from build123d import *

# Parameters (mm, degrees)
F1_DEPTH = 76.2
F2_T     = -2.54


with BuildPart() as f1:
    # F0 (on Top) → F1 (new body)
    with BuildSketch(Plane.XY):
        Polygon((43.9940905122, 25.4), (21.9970452561, 12.7), (21.9970452561, -12.7), (43.9940905122, -25.4), (65.9911357684, -12.7), (65.9911357684, 12.7), align=None)
        Polygon((0, 25.4), (21.9970452561, 12.7), (43.9940905122, 25.4), (43.994090537, 50.8000000143), (21.9970452561, 63.5000000285), (-2.47e-08, 50.8000000143), align=None)
        Polygon((43.9940905122, -25.4), (21.9970452561, -12.7), (0, -25.4), (0, -50.8), (21.9970452561, -63.5), (43.9940905122, -50.8), align=None)
        Polygon((-21.9970452561, 12.7), (0, 25.4), (0, 50.8), (-21.9970452561, 63.5), (-43.9940905122, 50.8), (-43.9940905122, 25.4), align=None)
        Polygon((0, -50.8), (0, -25.4), (-21.9970452561, -12.7), (-43.9940905122, -25.4), (-43.9940905122, -50.8), (-21.9970452561, -63.5), align=None)
        Polygon((-21.9970452561, -12.7), (-21.9970452561, 12.7), (-43.9940905122, 25.4), (-65.9911357684, 12.7), (-65.9911357684, -12.7), (-43.9940905122, -25.4), align=None)
        Polygon((21.9970452561, -12.7), (21.9970452561, 12.7), (0, 25.4), (-21.9970452561, 12.7), (-21.9970452561, -12.7), (0, -25.4), align=None)
    extrude(amount=F1_DEPTH)

    # F2
    f2_openings = [f1.faces().sort_by_distance(p)[0] for p in [
        (0, 0, 76.2),
    ]]
    offset(amount=F2_T, openings=f2_openings, kind=Kind.INTERSECTION)


solid = f1.part
Geometry check sheet. Reference: the model listing, model coordinates, mm. A direction names the side the tool comes from. Round coordinates to 2 decimals unless told otherwise and drop trailing zeros. Loops run counter-clockwise (first coordinate to the right, second up) from the corner with the lowest first, then second, coordinate; pieces in that order, holes last. Notation, with made-up numbers: (20.5, -29.5) - (31.5, -29.5) arc R23 cw to (31.5, -5.5) - close; hole circle Ø2 at (7.5, 33). An arc over 180 degrees is marked (long way). One line per question, with ' | ' between items. Start each with the question number.
1. Scan lines: line 1 (X direction, y = 8, z = 13); line 2 (X direction, y = -46, z = 64); line 3 (Z direction, x = -11.5, y = -26.5). Record each from-to range of solid material in increasing order. Write a range as [from, to].
2. Draft check along Y on faces 1 (the face through (-33.15, -57.06, 37.57)), 2 (the face through (-52.3, 17.67, 38.85)), 3 (the face through (-43.994, -38, 38)). Enter one of: released by +Y, released by -Y, zero draft, split by the parting line, or undercut.
3. Depth check by flat-ended pin: pin 1 (12.5 mm diameter, centred on y = -33, z = 38.5, fed in from +X); pin 2 (4 mm diameter, centred on x = 30, y = 50, fed in from +Z); pin 3 (5 mm diameter, centred on x = 36.5, z = 64.5, fed in from +Y). Enter the tip coordinate at first touch or a pass-through.
4. Tool access check on faces 4 (the face through (-43.994, 38, 38)), 5 (the face through (-11.153, -57.239, 37.567)), 6 (the face through (-10.84, 57.06, 37.57)), 7 (the face through (55.15, 18.96, 37.57)), 8 (the face through (-11.153, -54.306, 38.854)). Record the directions out of +Z, -Z, +X, -X, +Y, -Y that give a thin tool (end or side, any length) a straight path to the whole face; none if there is none.
5. Cross-section at A-A on y = -4. Record the cut outline in (x, z), then the cut area to 3 significant figures.
6. Cross-section at B-B on x = 53.5. Record the cut outline in (y, z).
Taken from the geometry:
1) line 1: [-65.99, -63.45], [63.45, 65.99] | line 2: [-43.99, -41.45], [41.45, 43.99] | line 3: [0, 2.54]
2) face 1: released by -Y | face 2: undercut | face 3: zero draft
3) pin 1: x = 43.99 | pin 2: z = 2.54 | pin 3: y = 56.57
4) face 4: +Z, -Z, -X, +Y | face 5: +Z, -Z, -Y | face 6: +Z, -Z, +Y | face 7: +Z, -Z, +X, +Y | face 8: +Z
5) outline: (-65.99, 0) - (65.99, 0) - (65.99, 76.2) - (63.45, 76.2) - (63.45, 2.54) - (-63.45, 2.54) - (-63.45, 76.2) - (-65.99, 76.2) - close | area: 709 mm²
6) outline: (-19.91, 0) - (19.91, 0) - (19.91, 76.2) - (16.98, 76.2) - (16.98, 2.54) - (-16.98, 2.54) - (-16.98, 76.2) - (-19.91, 76.2) - close
